Could you check a few things on this model? Use its own coordinates, in mm. Round coordinates to 2 decimals unless told otherwise and drop trailing zeros. Loops run counter-clockwise (first coordinate to the right, second up) from the corner with the lowest first, then second, coordinate; pieces in that order, holes last. Notation, with made-up numbers: M 39,58.25 L 45,58.25 A19 ccw 45,64.25 Z; hole C 82,20 d11. An arc over 180 degrees is marked long. Return JSON: item names as keys, results as strings. Group by question number.
```python
from build123d import *

# Parameters (mm, degrees)
BOX_W          = 508
BOX_H          = 50.8
BOX_DEPTH      = 6.35
BOX_ROLL_ANGLE = -45


with BuildPart() as part:
    # Box → Box (new body)
    with BuildSketch(Plane.XY):
        with Locations((254, 25.4)):
            Rectangle(BOX_W, BOX_H)
    extrude(amount=BOX_DEPTH)


with BuildPart() as part_1:
    # Box roll: moved
    add(part.part.rotate(Axis((0, 0, 0), (1, 0, 0)), BOX_ROLL_ANGLE))


with BuildPart() as part_2:
    # Box placement: moved
    add(part_1.part.moved(Location((-12.7, 0, 0))))


solid = part_2.part
```
1. If we section it at A-A, the plane x = 395: Please give me the cut outline in (y, z).
2. If we section it at B-B, the plane z = -13.5: Please give me the cut outline in (x, y), then the cut area to 3 significant figures.
3. I need wall thicknesses on probe 1 along Y at (x, z) = (86.5, -19); probe 2 along Y at (x, z) = (238, -11.5); probe 3 along Z at (x, y) = (376.5, 15.5). Which ranges of each line are inside material? Lowest first, please.
4. I'm going to push flat-ended pins straight in: pin 1 Ø2 at (x, z) = (45.5, -22) entering from -Y; pin 2 Ø5 at (x, z) = (411.5, -1.5) entering from +Y; pin 3 Ø5 at (x, y) = (374.5, 10.5) entering from -Z; pin 4 Ø5 at (y, z) = (11, -12) entering from -X. Where does each tip first touch, or does it pass through?
Geometry results:
{
 "1": {"outline": "M 0,0 L 35.92,-35.92 L 40.41,-31.43 L 4.49,4.49 Z"},
 "2": {"outline": "M -12.7,13.5 L 495.3,13.5 L 495.3,22.48 L -12.7,22.48 Z", "area": "4,560 mm^2"},
 "3": {"probe 1": "19 to 27.98", "probe 2": "11.5 to 20.48", "probe 3": "-15.5 to -6.52"},
 "4": {"pin 1": "y = 21", "pin 2": "y = 12.98", "pin 3": "z = -13", "pin 4": "x = -12.7"}
}
